Could you check a few things on this model? Use its own coordinates, in mm. Give positions to 0.01 mm unless a question says otherwise; leave off trailing zeros. Write each loop counter-clockwise with the first axis right and the second up, starting at its lowest first coordinate (ties: lowest second). Pieces come first, ordered by that corner, then holes. Notation, with made-up numbers: (-13, 5.5) - (30, 5.5) arc R19 ccw to (30, 28.5) - close; hole circle Ø8 at (23, -20). An arc over 180 degrees is marked (long way). Use one line per item in the form item = value.
```python
from build123d import *

# Parameters (mm, degrees)
CROQUIS1_R              = 1.1
CROQUIS1_R_2            = 3
SALIENTE_EXTRUIR1_DEPTH = 2
CORTAR_EXTRUIR1_START   = -2
CORTAR_EXTRUIR1_DEPTH   = 2
CROQUIS3_R              = 5
CORTAR_EXTRUIR2_DEPTH   = 2


with BuildPart() as part:
    # Croquis1 → Saliente-Extruir1 (new body)
    with BuildSketch(Plane.XY):
        with BuildLine():
            Line((-64.740473431, 32.731866916), (-64.740473431, 13.131866916))
            ThreePointArc((-64.740473431, 13.131866916), (-63.949661741, 11.222678607), (-62.040473431, 10.431866916))
            Line((-62.040473431, 10.431866916), (-42.440473431, 10.431866916))
            ThreePointArc((-42.440473431, 10.431866916), (-40.531285122, 11.222678607), (-39.740473431, 13.131866916))
            Line((-39.740473431, 13.131866916), (-39.740473431, 32.731866916))
            ThreePointArc((-39.740473431, 32.731866916), (-40.531285122, 34.641055225), (-42.440473431, 35.431866916))
            Line((-42.440473431, 35.431866916), (-62.040473431, 35.431866916))
            ThreePointArc((-62.040473431, 35.431866916), (-63.949661741, 34.641055225), (-64.740473431, 32.731866916))
        make_face()
        with Locations((-45.16940562, 30.002934728)):
            Circle(CROQUIS1_R, mode=Mode.SUBTRACT)
        with Locations((-52.240473431, 22.931866916)):
            Circle(CROQUIS1_R_2, mode=Mode.SUBTRACT)
        with Locations((-45.16940562, 15.860799104)):
            Circle(CROQUIS1_R, mode=Mode.SUBTRACT)
        with Locations((-59.311541243, 15.860799104)):
            Circle(CROQUIS1_R, mode=Mode.SUBTRACT)
        with Locations((-59.311541243, 30.002934728)):
            Circle(CROQUIS1_R, mode=Mode.SUBTRACT)
    extrude(amount=SALIENTE_EXTRUIR1_DEPTH)

    # Croquis2 → Cortar-Extruir1 (cut)
    with BuildSketch(Plane.XY.offset(2).offset(CORTAR_EXTRUIR1_START)):
        with BuildLine():
            Line((-64.740473431, 32.731866916), (-64.740473431, 13.131866916))
            ThreePointArc((-64.740473431, 13.131866916), (-63.949661741, 11.222678607), (-62.040473431, 10.431866916))
            Line((-62.040473431, 10.431866916), (-42.440473431, 10.431866916))
            ThreePointArc((-42.440473431, 10.431866916), (-40.531285122, 11.222678607), (-39.740473431, 13.131866916))
            Line((-39.740473431, 13.131866916), (-39.740473431, 32.731866916))
            ThreePointArc((-39.740473431, 32.731866916), (-40.531285122, 34.641055225), (-42.440473431, 35.431866916))
            Line((-42.440473431, 35.431866916), (-62.040473431, 35.431866916))
            ThreePointArc((-62.040473431, 35.431866916), (-63.949661741, 34.641055225), (-64.740473431, 32.731866916))
        make_face()
        with BuildLine():
            Line((-64.390473431, 32.731866916), (-64.390473431, 13.131866916))
            ThreePointArc((-64.390473431, 13.131866916), (-63.702174367, 11.47016598), (-62.040473431, 10.781866916))
            Line((-62.040473431, 10.781866916), (-42.440473431, 10.781866916))
            ThreePointArc((-42.440473431, 10.781866916), (-40.778772496, 11.47016598), (-40.090473431, 13.131866916))
            Line((-40.090473431, 13.131866916), (-40.090473431, 32.731866916))
            ThreePointArc((-40.090473431, 32.731866916), (-40.778772496, 34.393567852), (-42.440473431, 35.081866916))
            Line((-42.440473431, 35.081866916), (-62.040473431, 35.081866916))
            ThreePointArc((-62.040473431, 35.081866916), (-63.702174367, 34.393567852), (-64.390473431, 32.731866916))
        make_face(mode=Mode.SUBTRACT)
    extrude(amount=CORTAR_EXTRUIR1_DEPTH, mode=Mode.SUBTRACT)

    # Croquis3 → Cortar-Extruir2 (cut)
    with BuildSketch(Plane.XY.offset(2)):
        with Locations((-52.240473431, 22.931866916)):
            Circle(CROQUIS3_R)
    extrude(amount=-CORTAR_EXTRUIR2_DEPTH, mode=Mode.SUBTRACT)


solid = part.part
```
1. Imagine slicing it at C-C, the plane x = -55.75. List the corners of the cut face in (y, z) for me.
Response values:
outline = (10.78, 0) - (19.37, 0) - (19.37, 2) - (10.78, 2) - close; (26.49, 0) - (35.08, 0) - (35.08, 2) - (26.49, 2) - close
2. If we mould it in two halves opening along Y, with no side actions, what happens to faces 1 (the face through (-52.4, 17.7, 0)), 2 (the face through (-40.8, 11.45, 0.99)), 3 (the face through (-58.26, 16.19, 0.99))? For each: pulls with the +Y half, pulls with the -Y half, needs draft (parallel to the pull), parting line crosses it, or undercut.
Response values:
face_1 = needs draft
face_2 = pulls with the -Y half
face_3 = undercut
3. Imagine slicing it at D-D, the plane y = 15.5. List the corners of the cut face in (x, z) for me.
Response values:
outline = (-64.39, 0) - (-60.35, 0) - (-60.35, 2) - (-64.39, 2) - close; (-58.27, 0) - (-46.21, 0) - (-46.21, 2) - (-58.27, 2) - close; (-44.13, 0) - (-40.09, 0) - (-40.09, 2) - (-44.13, 2) - close
4. Imagine slicing it at A-A, the plane x = -58.75. List the corners of the cut face in (y, z) for me.
Response values:
outline = (10.78, 0) - (14.91, 0) - (14.91, 2) - (10.78, 2) - close; (16.81, 0) - (29.06, 0) - (29.06, 2) - (16.81, 2) - close; (30.95, 0) - (35.08, 0) - (35.08, 2) - (30.95, 2) - close
5. Imagine slicing it at B-B, the plane y = 20.5. List the corners of the cut face in (x, z) for me.
Response values:
outline = (-64.39, 0) - (-56.61, 0) - (-56.61, 2) - (-64.39, 2) - close; (-47.87, 0) - (-40.09, 0) - (-40.09, 2) - (-47.87, 2) - close
6. For pin 1 (1.3 mm diameter, centred on x = -45.17, y = 15.86, fed in from -Z), with a flat end and sliding along its axis, tell me the tip position at first contact or that it passes through.
Response values:
pin_1 = through
7. If I drill on line 1 (Y direction, x = -45.75, z = 0.25); line 2 (Y direction, x = -60.25, z = 1.2); line 3 (X direction, y = 21.25, z = 1.85), over which ranges is the centre line in solid material (lowest first)? Write a range as from..to.
Response values:
line_1 = 10.78..14.93, 16.8..29.07, 30.94..35.08
line_2 = 10.78..15.29, 16.43..29.43, 30.58..35.08
line_3 = -64.39..-56.95, -47.53..-40.09
